Check sheet for the modelled part. Datum: model origin and axes. Units: mm. Face numbers are marked on the shaded views. A direction names the side the tool comes from. Round coordinates to 2 decimals unless told otherwise and drop trailing zeros. Order: outer loops, then holes, each group sorted by start corner. A loop starts at its lowest first (then second) coordinate and runs counter-clockwise, first axis right, second up.
(1) Sectioned sample at C-C, the plane z = 301. Enter the section's corners in (x, y).
(2) Depth check by flat-ended pin: pin 1 (1.5 mm diameter, centred on y = -49, z = 116.5, fed in from -X); pin 2 (1.5 mm diameter, centred on x = -14.5, y = 102, fed in from -Z); pin 3 (15 mm diameter, centred on y = 103, z = -118, fed in from -X). Enter the tip coordinate at first touch or a pass-through.
(3) Sectioned sample at A-A, the plane y = 0. Enter the section's corners in (x, z), and give its area (3 significant figures).
(4) Tool access check on the marked faces 1, 2, 3 and 4. Record the directions out of +Z, -Z, +X, -X, +Y, -Y that give a thin tool (end or side, any length) a straight path to the whole face; none if there is none.
(5) Mould release check, pull along Y, two halves, no side actions. Record for the marked faces 5, 6 and 7: released by +Y, released by -Y, zero draft, split by the parting line, or undercut.
(6) Sectioned sample at B-B, the plane z = 35.5. Enter the section's corners in (x, y).
(7) Thickness scan on probe 1 along Y at (x, z) = (419, 166); probe 2 along X at (y, z) = (133, -94); probe 3 along Z at (x, y) = (499, 101.5). Record the ranges inside material, lowest first.
(8) Sectioned sample at D-D, the plane y = -124. Enter the section's corners in (x, z), and give its area (3 significant figures).
```python
from build123d import *

# Parameters (mm, degrees)
F1_DEPTH = 300
F2_W     = 1700
F2_H     = 480
F3_DEPTH = 364.080291
F4_W     = 1700
F4_H     = 480
F5_DEPTH = 100
F6_W     = 550
F6_H     = 480
F7_DEPTH = 50
F9_DEPTH = 300.001
F10_R    = 50


with BuildPart() as f1:
    # F0 (on Front) → F1 (new body, symmetric)
    with BuildSketch(Plane.XZ):
        with BuildLine():
            Line((-350, 0), (0, 0))
            Line((0, 0), (350, 0))
            Line((350, 0), (350, -150))
            Line((350, -150), (700, -150))
            Line((700, -150), (700, -50))
            Line((700, -50), (850, -50))
            Line((850, -50), (850, 100))
            ThreePointArc((850, 100), (0, 364.079291), (-850, 100))
            Line((-850, 100), (-850, -50))
            Line((-850, -50), (-700, -50))
            Line((-700, -50), (-700, -150))
            Line((-700, -150), (-350, -150))
            Line((-350, -150), (-350, 0))
        make_face()
    extrude(amount=F1_DEPTH, both=True)

    # F2 (on Top) → F3 (cut, through all)
    with BuildSketch(Plane.XY):
        Rectangle(F2_W, F2_H)
    extrude(amount=F3_DEPTH, mode=Mode.SUBTRACT)

    # F4 (on face) → F5 (join)
    with BuildSketch(Plane.XY):
        Rectangle(F4_W, F4_H)
    extrude(amount=F5_DEPTH)

    # F6 (on face) → F7 (join)
    with BuildSketch(Plane.XY.offset(100)):
        Rectangle(F6_W, F6_H)
    extrude(amount=F7_DEPTH)

    # F8 (on face) → F9 (cut, through all)
    with BuildSketch(Plane.XY.offset(150)):
        with BuildLine():
            Line((-100, -100), (100, -100))
            ThreePointArc((100, -100), (200, 0), (100, 100))
            Line((100, 100), (-100, 100))
            ThreePointArc((-100, 100), (-200, 0), (-100, -100))
        make_face()
    extrude(amount=-F9_DEPTH, mode=Mode.SUBTRACT)

    # F10
    f10_edges = [f1.edges().sort_by_distance(p)[0] for p in [
        (-350, 0, 0),
        (350, 0, 0),
        (-700, 0, -50),
        (700, 0, -50),
    ]]
    fillet(f10_edges, radius=F10_R)


solid = f1.part
```
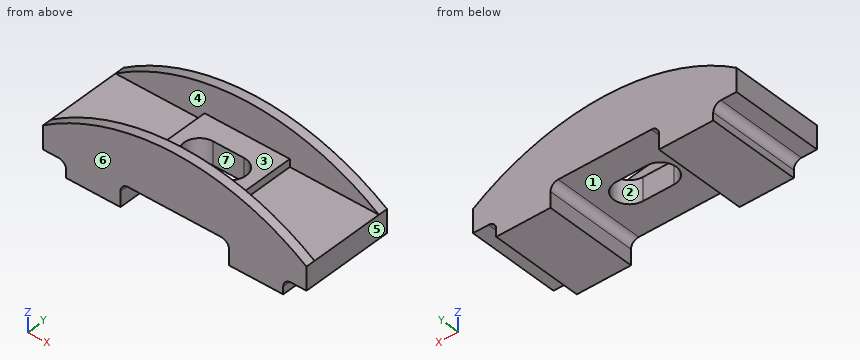
Derived:
1. outline: (-430.42, -300) - (430.42, -300) - (430.42, -240) - (-430.42, -240) - close; (-430.42, 240) - (430.42, 240) - (430.42, 300) - (-430.42, 300) - close
2. pin 1: stops at x = -275
2. pin 2: stops at z = 0
2. pin 3: stops at x = -700
3. outline: (-850, -50) - (-750, -50) arc R50 cw to (-700, -100) - (-700, -150) - (-350, -150) - (-350, -50) arc R50 cw to (-300, 0) - (-200, 0) - (-200, 150) - (-275, 150) - (-275, 100) - (-850, 100) - close; (200, 0) - (300, 0) arc R50 cw to (350, -50) - (350, -150) - (700, -150) - (700, -100) arc R50 cw to (750, -50) - (850, -50) - (850, 100) - (275, 100) - (275, 150) - (200, 150) - close
3. area: 260,000 mm2
4. face 1: -Z, +Y, -Y
4. face 2: +Z, -Z
4. face 3: +Z, +X, -X
4. face 4: +Z
5. face 5: zero draft
5. face 6: released by -Y
5. face 7: undercut
6. outline: (-850, -300) - (850, -300) - (850, 300) - (-850, 300) - close; hole (-100, -100) - (100, -100) arc R100 ccw to (100, 100) - (-100, 100) arc R100 ccw to start
7. probe 1: y = -300 to -240, 240 to 300
7. probe 2: x = -700.36 to -350, 350 to 700.36
7. probe 3: z = -150 to 100
8. outline: (-850, -50) - (-750, -50) arc R50 cw to (-700, -100) - (-700, -150) - (-350, -150) - (-350, -50) arc R50 cw to (-300, 0) - (300, 0) arc R50 cw to (350, -50) - (350, -150) - (700, -150) - (700, -100) arc R50 cw to (750, -50) - (850, -50) - (850, 100) - (275, 100) - (275, 150) - (-275, 150) - (-275, 100) - (-850, 100) - close
8. area: 320,000 mm2
